Job drawing, mm, ordinate dimensions from the low corner. One solid piece. A direction names the side the tool comes from. Give positions to 0.01 mm unless a question says otherwise; leave off trailing zeros. Loops run counter-clockwise (first coordinate to the right, second up) from the corner with the lowest first, then second, coordinate; pieces in that order, holes last. Notation, with made-up numbers: (17.5, 26) - (64.5, 26) arc R27 cw to (64.5, 53) - close; hole circle Ø8 at (6.25, -11.75). An arc over 180 degrees is marked (long way). Use a Markdown table: item, result.
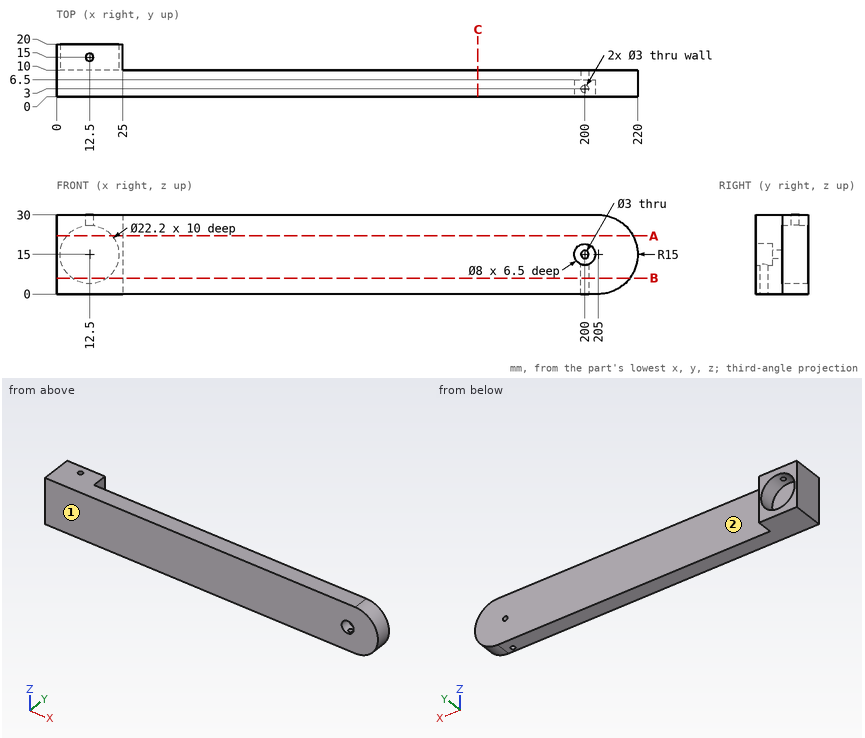
(1) Slice it at C-C, the plane x = 159.5. Write the cut outline in (y, z), plus the area to 3 significant figures.
Computed:
| item | result |
|---|---|
| outline | (0, 0) - (10, 0) - (10, 30) - (0, 30) - close |
| area | 300 mm² |
(2) Slice it at B-B, the plane z = 6. Write the cut outline in (x, y).
Computed:
| item | result |
|---|---|
| outline | (0, 0) - (217, 0) - (217, 10) - (25, 10) - (25, 20) - (19, 20) - (19, 10) - (6, 10) - (6, 20) - (0, 20) - close; hole circle Ø3 at (200, 3) |
(3) Slice it at A-A, the plane z = 22. Write the cut outline in (x, y).
Computed:
| item | result |
|---|---|
| outline | (0, 0) - (218.27, 0) - (218.27, 10) - (25, 10) - (25, 20) - (21.11, 20) - (21.11, 10) - (3.89, 10) - (3.89, 20) - (0, 20) - close |
(4) Drill centre lines: probe 1 along Y at (x, z) = (200, 8); probe 2 along X at (y, z) = (12.5, 15); probe 3 along X at (y, z) = (1.5, 15). Where is each one in solid material? Low to high. Write a range as [from, to].
Computed:
| item | result |
|---|---|
| probe 1 | [0, 1.5], [4.5, 10] |
| probe 2 | [0, 1.4], [23.6, 25] |
| probe 3 | [0, 196], [204, 220] |
(5) 3-axis set-ups, long thin cutter, end or side, ignore diameter. For the marked faces 1 and 2: which of +Z, -Z, +X, -X, +Y, -Y reach the whole face in a straight line?
Computed:
| item | result |
|---|---|
| face 1 | +Z, -Z, +X, -X, -Y |
| face 2 | +Z, -Z, +X, +Y |
(6) Pin check, flat tips, straight feed: P1, Ø1.8, axis at x = 200, y = 3, coming from the -Z side; P2, Ø9, axis at x = 200, z = 15, coming from the +Y side; P3, Ø4, axis at y = 17.5, z = 11.5, coming from the +X side; P4, Ø8, axis at x = 70.5, y = 16.5, coming from the -Z side (1 decimal). Stop position of each tip, or through.
Computed:
| item | result |
|---|---|
| P1 | z = 18.9 |
| P2 | y = 10 |
| P3 | x = 25 |
| P4 | through |
